from build123d import *

# Parameters (mm, degrees)
SKETCH1_R           = 3.5
BOSS_EXTRUDE1_DEPTH = 4
CUT_EXTRUDE1_DEPTH  = 2.25
CHAMFER1_SIZE       = 0.35


with BuildPart() as part:
    # Sketch1 → Boss-Extrude1 (new body)
    with BuildSketch(Plane(origin=(0, 0, 0), x_dir=(1, 0, 0), z_dir=(0, 1, 0))):
        with Locations(Location((0, 0, 0), (0, 0, 270))):
            Circle(SKETCH1_R)
    extrude(amount=BOSS_EXTRUDE1_DEPTH)

    # Sketch2 → Cut-Extrude1 (cut)
    with BuildSketch(Plane(origin=(0, 4, 0), x_dir=(1, 0, 0), z_dir=(0, 1, 0))):
        Polygon((0.866025404, 1.5), (-0.866025404, 1.5), (-1.732050808, 0), (-0.866025404, -1.5), (0.866025404, -1.5), (1.732050808, 0), align=None)
    extrude(amount=-CUT_EXTRUDE1_DEPTH, mode=Mode.SUBTRACT)

    # Cut-Extrude2 cone 1 section (through the dimple's axis) → Cut-Extrude2 (revolve, cut)
    with BuildSketch(Plane(origin=(0, 4, 0), x_dir=(0, 0, 1), z_dir=(1, 0, 0))):
        Polygon((0, 0), (1.732050808, 0), (0, 1.732050808), align=None)
    revolve(axis=Axis((0, 4, 0), (0, -1, 0)), mode=Mode.SUBTRACT)

    # Chamfer1
    chamfer1_edges = [part.edges().sort_by_distance(p)[0] for p in [
        (0, 0, -3.5),
        (0, 4, -3.5),
    ]]
    chamfer(chamfer1_edges, length=CHAMFER1_SIZE)


solid = part.part
Input: part model. Units: mm. Frame: model coordinates. A direction names the side the tool comes from. Coordinates: 2 decimals unless noted, no trailing zeros. Write each loop counter-clockwise with the first axis right and the second up, starting at its lowest first coordinate (ties: lowest second). Pieces come first, ordered by that corner, then holes. Notation, with made-up numbers: M 11.5,-40 L 60.5,-40 A21 cw 60.5,-6 Z; hole C 36.5,83 d1. An arc over 180 degrees is marked long. Answer as a JSON object with one key per item and string values. Group by question number.
(1) Section B-B on x = 0. Output: boundary loops of the cut face in (y, z).
(2) Ray query, line 1 along X through (y, z) = (2.6, -0.25); line 2 along Z through (x, y) = (-1.5, 3.5); line 3 along Z through (x, y) = (1, 2.55). Return the intervals inside material, ascending. Write a range as [from, to].
(3) Set-up query: faces 1 (the face through (-1.4, 4, 1.4)), 2 (the face through (1.39, 3.88, -0.82)). Return all of +Z, -Z, +X, -X, +Y, -Y with unobstructed straight access to the full face (end or side cutting, diameter ignored); none if empty.
(4) Mould query, pull axis Z, two halves, no side actions, for faces 3 (the face through (0, 3, -1.5)), 4 (the face through (-3.417, 1.977, -0.759)), 5 (the face through (0, 0, 0)). Classes: pulls with the +Z half, pulls with the -Z half, needs draft (parallel to the pull), parting line crosses it, or undercut.
(5) Section A-A on y = 2.55. Output: boundary loops of the cut face in (x, z), plus the area to 3 significant figures.
(6) Contact query for a flat-ended pin moving along its axis: P1, Ø0.9, axis at x = 0.5, y = 3.5, coming from the -Z side. Output: stop coordinate, or through.
(7) Section C-C on y = 0.85. Output: boundary loops of the cut face in (x, z).
Result set:
{
 "1": {"outline": "M 0,-3.15 L 0.35,-3.5 L 3.65,-3.5 L 4,-3.15 L 4,-1.73 L 3.77,-1.5 L 1.75,-1.5 L 1.75,1.5 L 3.77,1.5 L 4,1.73 L 4,3.15 L 3.65,3.5 L 0.35,3.5 L 0,3.15 Z"},
 "2": {"line 1": "x = [-3.49, -1.59], [1.59, 3.49]", "line 2": "z = [-3.16, -0.4], [0.4, 3.16]", "line 3": "z = [-3.35, -1.27], [1.27, 3.35]"},
 "3": {"face 1": "+Z, -Z, +X, -X, +Y", "face 2": "+Y"},
 "4": {"face 3": "undercut", "face 4": "parting line crosses it", "face 5": "needs draft"},
 "5": {"outline": "C 0,0 d7; hole M -1.73,0 L -0.87,-1.5 L 0.87,-1.5 L 1.73,0 L 0.87,1.5 L -0.87,1.5 Z", "area": "30.7 mm2"},
 "6": {"P1": "stops at z = -3.5"},
 "7": {"outline": "C 0,0 d7"}
}
